Here's how the part is built. I have some questions about the finished solid (model axes, mm). A direction names the side the tool comes from. Coordinates: 2 decimals unless noted, no trailing zeros. Loops run counter-clockwise (first coordinate to the right, second up) from the corner with the lowest first, then second, coordinate; pieces in that order, holes last.
from build123d import *

# Parameters (mm, degrees)
F1_DEPTH = 7.62
F3_T     = -2.286
F5_DEPTH = 15.5702
F6_R     = 1.27


with BuildPart() as f1:
    # F0 (on Front) → F1 (new body)
    with BuildSketch(Plane.XZ):
        with BuildLine():
            Line((23.2504412389, 63.8689214671), (-24.1253591931, 63.8689214671))
            ThreePointArc((-24.1253591931, 63.8689214671), (-30.4115384778, 61.2651007518), (-33.0153591931, 54.9789214671))
            Line((-33.0153591931, 54.9789214671), (-33.0153591931, -67.0640870786))
            ThreePointArc((-33.0153591931, -67.0640870786), (-30.4115384778, -73.3502663633), (-24.1253591931, -75.9540870786))
            Line((-24.1253591931, -75.9540870786), (23.2504412389, -75.9540870786))
            ThreePointArc((23.2504412389, -75.9540870786), (29.5366205236, -73.3502663633), (32.1404412389, -67.0640870786))
            Line((32.1404412389, -67.0640870786), (32.1404412389, 54.9789214671))
            ThreePointArc((32.1404412389, 54.9789214671), (29.5366205236, 61.2651007518), (23.2504412389, 63.8689214671))
        make_face()
    extrude(amount=F1_DEPTH)

    # F3
    f3_openings = [f1.faces().sort_by_distance(p)[0] for p in [
        (-0.437459, -7.62, -6.042583),
    ]]
    offset(amount=F3_T, openings=f3_openings)

    # F4 (on face) → F5 (cut)
    with BuildSketch(Plane.XY.offset(63.8689214671)):
        with BuildLine():
            Line((3.8106236157, -2.5396881921), (-3.81, -2.5396881921))
            ThreePointArc((-3.81, -2.5396881921), (-4.7080256121, -2.91166258), (-5.08, -3.8096881921))
            Line((-5.08, -3.8096881921), (-5.08, -3.8103118079))
            ThreePointArc((-5.08, -3.8103118079), (-4.7080256121, -4.70833742), (-3.81, -5.0803118079))
            Line((-3.81, -5.0803118079), (3.8106236157, -5.0803118079))
            ThreePointArc((3.8106236157, -5.0803118079), (4.7086492278, -4.70833742), (5.0806236157, -3.8103118079))
            Line((5.0806236157, -3.8103118079), (5.0806236157, -3.8096881921))
            ThreePointArc((5.0806236157, -3.8096881921), (4.7086492278, -2.91166258), (3.8106236157, -2.5396881921))
        make_face()
    extrude(amount=-F5_DEPTH, mode=Mode.SUBTRACT)

    # F6
    f6_edges = [f1.edges().sort_by_distance(p)[0] for p in [
        (-0.437459, -7.62, -75.954087),
        (29.536621, -7.62, -73.350266),
        (32.140441, -7.62, -6.042583),
        (29.536621, -7.62, 61.265101),
        (-0.437459, -7.62, 63.868921),
        (-30.411538, -7.62, -73.350266),
        (-33.015359, -7.62, -6.042583),
    ]]
    fillet(f6_edges, radius=F6_R)


solid = f1.part
Q1. Suppose I cut it at A-A on x = -2. Write out the boundary of the cut face in (y, z).
Q2. For faces 4 (the cylindrical face through (29.467, -3.131, -73.419)), 5 (the cylindrical face through (-28.743, -4.916, 59.7)), which set-ups out of +Z, -Z, +X, -X, +Y, -Y let a thin tool reach every point of the face, with its end or its side?
Q3. Please list where these lines run through material, in increasing order: probe 1 along Z at (x, y) = (-18.5, -6.5); probe 2 along Z at (x, y) = (0.5, -2.5); probe 3 along X at (y, z) = (-4.5, 6).
Q4. We'd pull the mould along X, two halves only. Please class faces 1 (the flat face through (-33.015, -3, -5)), 2 (the flat face through (-30.729, -5, -5)), 3 (the cylindrical face through (29.6, -3.1, 61.2)): pulls with the +X half, pulls with the -X half, needs draft (parallel to the pull), parting line crosses it, or undercut.
Q5. Suppose I cut it at B-B on z = 35.5. Write out the boundary of the cut face in (x, y), and give its area (3 significant figures).
Q6. Will this pin go through, and if not, where does the flat tip stop? P1, Ø3, axis at x = 10, z = 32.5, coming from the -Y side.
Check values:
1. outline: (-7.62, -74.68) arc R1.27 ccw to (-6.35, -75.95) - (0, -75.95) - (0, 63.87) - (-2.54, 63.87) - (-2.54, 61.58) - (-2.29, 61.58) - (-2.29, -73.67) - (-7.62, -73.67) - close; (-7.62, 61.58) - (-5.08, 61.58) - (-5.08, 63.87) - (-6.35, 63.87) arc R1.27 ccw to (-7.62, 62.6) - close
2. face 4: -Z, +X, +Y, -Y
2. face 5: -Y
3. probe 1: z = -75.95 to -73.67, 61.58 to 63.86
3. probe 2: z = -75.95 to -73.67, 61.58 to 63.87
3. probe 3: x = -33.02 to -30.73, 29.85 to 32.14
4. face 1: pulls with the -X half
4. face 2: undercut
4. face 3: pulls with the +X half
5. outline: (-33.02, -6.35) arc R1.27 ccw to (-31.75, -7.62) - (-30.73, -7.62) - (-30.73, -2.29) - (29.85, -2.29) - (29.85, -7.62) - (30.87, -7.62) arc R1.27 ccw to (32.14, -6.35) - (32.14, 0) - (-33.02, 0) - close
5. area: 173 mm2
6. P1: stops at y = -2.29
